```python
from build123d import *

# Parameters (mm, degrees)
F0_W     = 152.4
F0_H     = 152.4
F1_DEPTH = 152.4
F2_R     = 25.4
F3_DEPTH = 152.401


with BuildPart() as f1:
    # F0 (on Right) → F1 (new body)
    with BuildSketch(Plane.YZ):
        with Locations((76.2, -76.2)):
            Rectangle(F0_W, F0_H)
    extrude(amount=F1_DEPTH)

    # F2 (on face) → F3 (cut, through all)
    with BuildSketch(Plane.XY):
        with Locations((75.516477, 77.730492)):
            Circle(F2_R)
    extrude(amount=-F3_DEPTH, mode=Mode.SUBTRACT)


solid = f1.part
```
Geometry: final body of the model. Coordinates: model frame, mm. Give positions to 0.01 mm unless a question says otherwise; leave off trailing zeros. Loops run counter-clockwise (first coordinate to the right, second up) from the corner with the lowest first, then second, coordinate; pieces in that order, holes last. Notation, with made-up numbers: (11.25, 28) -> (39.25, 28) arc R20 cw to (39.25, 43) -> close; hole circle Ø11 at (20, 43.5). An arc over 180 degrees is marked (long way). Return JSON: item names as keys, results as strings.
Item 1: Mould query, pull axis X, two halves, no side actions, for faces 1 (the cylindrical face through (55.36, 62.275, -75.133)), 2 (the flat face through (75, 0, -77)), 3 (the flat face through (152.4, 75, -75)). Classes: released by +X, released by -X, zero draft, split by the parting line, or undercut.
Filled in:
{"face 1": "undercut", "face 2": "zero draft", "face 3": "released by +X"}
Item 2: Section A-A, the plane y = 72.5. Output: boundary loops of the cut face in (x, z), plus the area to 3 significant figures.
Filled in:
{"outline": "(0, -152.4) -> (50.66, -152.4) -> (50.66, 0) -> (0, 0) -> close; (100.37, -152.4) -> (152.4, -152.4) -> (152.4, 0) -> (100.37, 0) -> close", "area": "15,600 mm^2"}
Item 3: Section C-C, the plane z = -23. Output: boundary loops of the cut face in (x, y), plus the area to 3 significant figures.
Filled in:
{"outline": "(0, 0) -> (152.4, 0) -> (152.4, 152.4) -> (0, 152.4) -> close; hole circle Ø50.8 at (75.52, 77.73)", "area": "21,200 mm^2"}
Item 4: Section B-B, the plane x = 88. Output: boundary loops of the cut face in (y, z), plus the area to 3 significant figures.
Filled in:
{"outline": "(0, -152.4) -> (55.61, -152.4) -> (55.61, 0) -> (0, 0) -> close; (99.85, -152.4) -> (152.4, -152.4) -> (152.4, 0) -> (99.85, 0) -> close", "area": "16,500 mm^2"}
Item 5: Line query: line 1 (Y direction, x = 75.5, z = -98); line 2 (X direction, y = 93, z = -40); line 3 (Y direction, x = 73.5, z = -71.5). Output: solid intervals per line, ascending.
Filled in:
{"line 1": "0 to 52.33, 103.13 to 152.4", "line 2": "0 to 55.22, 95.81 to 152.4", "line 3": "0 to 52.41, 103.05 to 152.4"}
Item 6: Pin query (flat end, axial travel): P1, Ø10, axis at y = 94, z = -65.5, coming from the -X side. Return the tip coordinate at first contact, or that it passes through.
Filled in:
{"P1": "x = 0"}
